```python
from build123d import *

# Parameters (mm, degrees)
SKETCH_1_R                   = 15
EXTRUDE_1_DEPTH              = 30
SKETCH_2_W                   = 32
SKETCH_2_H                   = 45
EXTRUDE_2_DEPTH              = 10
HOLE_WIZARD_M4_1_D           = 4.5
HOLE_WIZARD_M4_1_CBORE_D     = 8
HOLE_WIZARD_M4_1_CBORE_DEPTH = 4
SKETCH_6_W                   = 78.990137636
SKETCH_6_H                   = 62.836735256
SKETCH_6_R                   = 25
CUT_EXTRUDE_1_DEPTH          = 30
SKETCH_7_R                   = 6
CUT_EXTRUDE_2_DEPTH          = 49.602983448


with BuildPart() as part:
    # 스케치1 → 보스-돌출1 (new body)
    with BuildSketch(Plane(origin=(0, 0, 0), x_dir=(1, 0, 0), z_dir=(0, 1, 0))):
        with Locations(Location((0, 0, 0), (0, 0, 270))):
            Circle(SKETCH_1_R)
    extrude(amount=EXTRUDE_1_DEPTH)

    # 스케치2 → 보스-돌출2 (add)
    with BuildSketch(Plane(origin=(0, 30, 0), x_dir=(1, 0, 0), z_dir=(0, 1, 0))):
        Rectangle(SKETCH_2_W, SKETCH_2_H)
    extrude(amount=EXTRUDE_2_DEPTH)

    # M4 소켓 머리 캡 나사용 카운터보어1 (through all)
    with Locations(Plane(origin=(0, 40, 0), x_dir=(1, 0, 0), z_dir=(0, 1, 0))):
        with Locations((-10, 17.320508076), (10, 17.320508076), (10, -17.320508076), (-10, -17.320508076)):
            CounterBoreHole(HOLE_WIZARD_M4_1_D / 2, HOLE_WIZARD_M4_1_CBORE_D / 2, HOLE_WIZARD_M4_1_CBORE_DEPTH)

    # 스케치6 → 컷-돌출1 (cut)
    with BuildSketch(Plane(origin=(0, 40, 0), x_dir=(1, 0, 0), z_dir=(0, 1, 0))):
        Rectangle(SKETCH_6_W, SKETCH_6_H)
        Circle(SKETCH_6_R, mode=Mode.SUBTRACT)
    extrude(amount=-CUT_EXTRUDE_1_DEPTH, mode=Mode.SUBTRACT)

    # 스케치7 → 컷-돌출2 (cut, through all)
    with BuildSketch(Plane(origin=(0, 40, 0), x_dir=(1, 0, 0), z_dir=(0, 1, 0))):
        with Locations(Location((0, 0, 0), (0, 0, 270))):
            Circle(SKETCH_7_R)
    extrude(amount=-CUT_EXTRUDE_2_DEPTH, mode=Mode.SUBTRACT)


solid = part.part
```
Check sheet for the modelled part. Datum: model origin and axes. Units: mm. A direction names the side the tool comes from. Give positions to 0.01 mm unless a question says otherwise; leave off trailing zeros. Write each loop counter-clockwise with the first axis right and the second up, starting at its lowest first coordinate (ties: lowest second). Pieces come first, ordered by that corner, then holes.
Item 1: Cross-section at C-C (x = -9). Enter the section's corners in (y, z), and give its area (3 significant figures).
Item 2: Draft check along X on faces 1 (the face through (-13.58, 35.07, 20.99)), 2 (the face through (10.29, 32.96, -19.55)), 3 (the face through (13.58, 35.07, -20.99)). Enter one of: released by +X, released by -X, zero draft, split by the parting line, or undercut.
Item 3: Gauge pin test, flat ends, axial feed: pin 1 (10 mm diameter, centred on x = -5, y = 17.5, fed in from +Z); pin 2 (2.5 mm diameter, centred on x = 10, z = 19, fed in from +Y); pin 3 (5 mm diameter, centred on x = 10, z = 17.32, fed in from -Y); pin 4 (9.5 mm diameter, centred on x = 0, z = 0, fed in from +Y). Record the tip position at first contact, or that the pin passes through.
Item 4: Cross-section at B-B (x = 0). Enter the section's corners in (y, z).
Item 5: Scan lines: L1, parallel to Z at x = 10, y = 37.75; L2, parallel to Z at x = 10, y = 32; L3, parallel to Y at x = 13.5, z = 15.5. Record each from-to range of solid material in increasing order.
Item 6: Cross-section at D-D (y = 34). Enter the section's corners in (x, z).
Item 7: Access from +Z, -Z, +X, -X, +Y, -Y to the whole of each face (thin tool, end or side, straight path). Record for faces 4 (the face through (-12.95, 38.03, 14.62)), 5 (the face through (16, 35, 0)), 6 (the face through (-14.45, 30, 4.69)).
Item 8: Cross-section at A-A (z = 0). Enter the section's corners in (x, y).
Report:
1. outline: (0, -12) - (30, -12) - (30, -15.3) - (36, -15.3) - (36, -13.45) - (40, -13.45) - (40, 13.45) - (36, 13.45) - (36, 15.3) - (30, 15.3) - (30, 12) - (0, 12) - close; (30, -22.5) - (40, -22.5) - (40, -21.19) - (36, -21.19) - (36, -19.34) - (30, -19.34) - close; (30, 19.34) - (36, 19.34) - (36, 21.19) - (40, 21.19) - (40, 22.5) - (30, 22.5) - close
1. area: 1,060 mm2
2. face 1: released by -X
2. face 2: undercut
2. face 3: released by +X
3. pin 1: stops at z = 15
3. pin 2: stops at y = 36
3. pin 3: stops at y = 30
3. pin 4: passes through
4. outline: (0, -15) - (30, -15) - (30, -22.5) - (40, -22.5) - (40, -6) - (0, -6) - close; (0, 6) - (40, 6) - (40, 22.5) - (30, 22.5) - (30, 15) - (0, 15) - close
5. L1: z = -22.5 to -21.32, -13.32 to 13.32, 21.32 to 22.5
5. L2: z = -22.5 to -19.57, -15.07 to 15.07, 19.57 to 22.5
5. L3: y = 30 to 36
6. outline: (-16, -19.21) arc R25 ccw to (-10.9, -22.5) - (10.9, -22.5) arc R25 ccw to (16, -19.21) - (16, 19.21) arc R25 ccw to (10.9, 22.5) - (-10.9, 22.5) arc R25 ccw to (-16, 19.21) - close; hole circle Ø4.5 at (-10, -17.32); hole circle Ø4.5 at (-10, 17.32); hole circle Ø12 at (0, 0); hole circle Ø4.5 at (10, -17.32); hole circle Ø4.5 at (10, 17.32)
7. face 4: +Y
7. face 5: +Z, -Z, +X, +Y, -Y
7. face 6: -Y
8. outline: (-16, 30) - (-15, 30) - (-15, 0) - (-6, 0) - (-6, 40) - (-16, 40) - close; (6, 0) - (15, 0) - (15, 30) - (16, 30) - (16, 40) - (6, 40) - close
